The model under review builds one solid part; all positions refer to its coordinate system, in mm. Coordinates: 2 decimals unless noted, no trailing zeros. Write each loop counter-clockwise with the first axis right and the second up, starting at its lowest first coordinate (ties: lowest second). Pieces come first, ordered by that corner, then holes. Notation, with made-up numbers: (-35, 9.25) - (14, 9.25) arc R17 ccw to (14, 40.25) - close; hole circle Ø8 at (81.25, 40.25). An arc over 180 degrees is marked (long way). Return JSON: item names as keys, results as strings. Group by question number.
(1) To check wall thickness, follow L1, parallel to Z at x = 15, y = 3.55; L2, parallel to X at y = 3.5, z = -130; L3, parallel to Z at x = -0.5, y = 3.55. State the ranges of each line that lie inside material, in increasing order. Write a range as from..to.
(2) Draft analysis for pull direction X (two halves, no side actions). For faces 1 (the face through (1.08, 2.96, 4.88)), 2 (the face through (25, 3, 2)), 3 (the face through (6, 6, 2)), state which applies: released by +X, released by -X, zero draft, split by the parting line, or undercut.
(3) We need section A-A on x = 0. State the section outline as (y, z) points, then the cut area to 3 significant figures.
Autodesk Inventor part; units mm, degrees
ref_plane "YZ Plane" through (0, 0, 0) normal (1, 0, 0) x (0, 1, 0)
ref_plane "XZ Plane" through (0, 0, 0) normal (0, 1, 0) x (-1, 0, 0)
ref_plane "XY Plane" through (0, 0, 0) normal (0, 0, 1) x (1, 0, 0)
sketch "Sketch1" plane through (0, 0, 0) normal (0, 1, 0) x (-1, 0, 0)
  circle A0 centre (0, 0) radius 5
  line L0 (25, 150) -> (-25, 150)
  line L1 (-25, 150) -> (-25, -150)
  line L2 (-25, -150) -> (25, -150)
  line L3 (25, -150) -> (25, 150)
  line L4 (25, 150) -> (-25, -150) construction
  line L5 (-25, 150) -> (25, -150) construction
  circle A1 centre (-15, 130) radius 1.5
  circle A2 centre (-15, -130) radius 1.5
  dimension "d0" = 10
  dimension "d6" = 50
  dimension "d7" = 300
  dimension "d15" = 3
  dimension "d16" = 10
  dimension "d17" = 3
  dimension "d20" = 20
  dimension "d21" = 20
extrude "Extrusion2" add sketch "Sketch1" along normal blind 6
equation "\"d21\" = d20"
properties part number "Estabilizador"
Ans:
{
 "1": {"L1": "-150..-131.5, -128.5..128.5, 131.5..150", "L2": "-25..13.5, 16.5..25", "L3": "-150..-4.97, 4.97..150"},
 "2": {"face 1": "undercut", "face 2": "released by +X", "face 3": "zero draft"},
 "3": {"outline": "(0, -150) - (6, -150) - (6, -5) - (0, -5) - close; (0, 5) - (6, 5) - (6, 150) - (0, 150) - close", "area": "1,740 mm²"}
}
